Build history of the part. All positions in model axes, mm. A direction names the side the tool comes from. Give positions to 0.01 mm unless a question says otherwise; leave off trailing zeros. Loops run counter-clockwise (first coordinate to the right, second up) from the corner with the lowest first, then second, coordinate; pieces in that order, holes last. Notation, with made-up numbers: (77, -33.75) - (106, -33.75) arc R21 ccw to (106, -6.75) - close; hole circle Ø6 at (47.25, 18). An arc over 180 degrees is marked (long way). Return JSON: item names as keys, results as strings. Group by question number.
1) 3-axis set-ups, long thin cutter, end or side, ignore diameter. For faces 4 (the face through (10, 0, 4)), 5 (the face through (9, 0, 4)): which of +Z, -Z, +X, -X, +Y, -Y reach the whole face in a straight line?
2) Drill centre lines: probe 1 along X at (y, z) = (-3.5, 120.5); probe 2 along X at (y, z) = (-9.25, -55) (3 decimals). Where is each one in solid material? Low to high. Write a range as from..to.
3) Slice it at A-A (z = 99). List the corners of the cut face in (x, y), and give its area (3 significant figures).
4) Drop flat-ended pins along their axis: pin 1 (2.5 mm diameter, centred on x = 0, z = -285, fed in from -Y); pin 2 (6.5 mm diameter, centred on x = 0, z = 55, fed in from +Y). Give the stop position or say it passes through.
5) Mould opens along X. For faces 1 (the face through (0, -9, 4)), 2 (the face through (-0.8, -9.6, -295)), 3 (the face through (-10, 0, 4)) say: released by +X, released by -X, zero draft, split by the parting line, or undercut.
```python
from build123d import *

# Parameters (mm, degrees)
SKETCH_1_W           = 20
SKETCH_1_H           = 20
SKETCH_1_W_2         = 18
SKETCH_1_H_2         = 18
EXTRUDE_1_DEPTH      = 295
SKETCH_2_R           = 2.025
CUT_EXTRUDE_1_DEPTH  = 45
SKETCH_3_R           = 3.8
CUT_EXTRUDE_2_DEPTH  = 5
SKETCH_4_R           = 2.025
CUT_EXTRUDE_3_DEPTH  = 73
SKETCH_15_R          = 2.025
CUT_EXTRUDE_14_DEPTH = 70


with BuildPart() as part:
    # 草图1 → 凸台-拉伸1 (new body, symmetric)
    with BuildSketch(Plane.XY):
        Rectangle(SKETCH_1_W, SKETCH_1_H)
        Rectangle(SKETCH_1_W_2, SKETCH_1_H_2, mode=Mode.SUBTRACT)
    extrude(amount=EXTRUDE_1_DEPTH, both=True)

    # 草图2 → 切除-拉伸1 (cut, symmetric)
    with BuildSketch(Plane(origin=(0, 10, 0), x_dir=(1, 0, 0), z_dir=(0, 1, 0))):
        with Locations((0, -75)):
            Circle(SKETCH_2_R)
        with Locations((0, -55)):
            Circle(SKETCH_2_R)
        with Locations((0, 55)):
            Circle(SKETCH_2_R)
        with Locations((0, 75)):
            Circle(SKETCH_2_R)
    extrude(amount=CUT_EXTRUDE_1_DEPTH, both=True, mode=Mode.SUBTRACT)

    # 草图3 → 切除-拉伸2 (cut, symmetric)
    with BuildSketch(Plane(origin=(0, 10, 0), x_dir=(1, 0, 0), z_dir=(0, 1, 0))):
        with Locations((0, 75)):
            Circle(SKETCH_3_R)
        with Locations((0, 55)):
            Circle(SKETCH_3_R)
        with Locations((0, -55)):
            Circle(SKETCH_3_R)
        with Locations((0, -75)):
            Circle(SKETCH_3_R)
    extrude(amount=CUT_EXTRUDE_2_DEPTH, both=True, mode=Mode.SUBTRACT)

    # 草图4 → 切除-拉伸3 (cut)
    with BuildSketch(Plane(origin=(10, 0, 0), x_dir=(0, 0, -1), z_dir=(1, 0, 0))):
        with Locations((-236, 0)):
            Circle(SKETCH_4_R)
        with Locations((-260.5, 0)):
            Circle(SKETCH_4_R)
        with Locations((-285, 0)):
            Circle(SKETCH_4_R)
    extrude(amount=-CUT_EXTRUDE_3_DEPTH, mode=Mode.SUBTRACT)

    # 草图15 → 切除-拉伸14 (cut)
    with BuildSketch(Plane.XZ.offset(10)):
        with Locations((0, 285)):
            Circle(SKETCH_15_R)
    cut_extrude_14 = extrude(amount=-CUT_EXTRUDE_14_DEPTH, mode=Mode.SUBTRACT)

    # 镜向2: 切除-拉伸14 across plane
    add(cut_extrude_14.mirror(Plane.XY), mode=Mode.SUBTRACT)


solid = part.part
```
Results:
{
 "1": {"face 4": "+Z, -Z, +X, +Y, -Y", "face 5": "+Z, -Z"},
 "2": {"probe 1": "-10..-9, 9..10", "probe 2": "-10..-2.025, 2.025..10"},
 "3": {"outline": "(-10, -10) - (10, -10) - (10, 10) - (-10, 10) - close; hole (-9, -9) - (9, -9) - (9, 9) - (-9, 9) - close", "area": "76.0 mm2"},
 "4": {"pin 1": "through", "pin 2": "y = -9"},
 "5": {"face 1": "undercut", "face 2": "zero draft", "face 3": "released by -X"}
}
